Drawing for the job (mm, zero at the part's lowest x, y, z). A direction names the side the tool comes from. Coordinates: 2 decimals unless noted, no trailing zeros. Order: outer loops, then holes, each group sorted by start corner. A loop starts at its lowest first (then second) coordinate and runs counter-clockwise, first axis right, second up. Notation, with made-up numbers: (-33.5, 32) - (1.5, 32) arc R33 ccw to (1.5, 67) - close; hole circle Ø4 at (-37.5, 26). An arc over 180 degrees is marked (long way). Put each result on its own line as item: value. Start each with the question number.
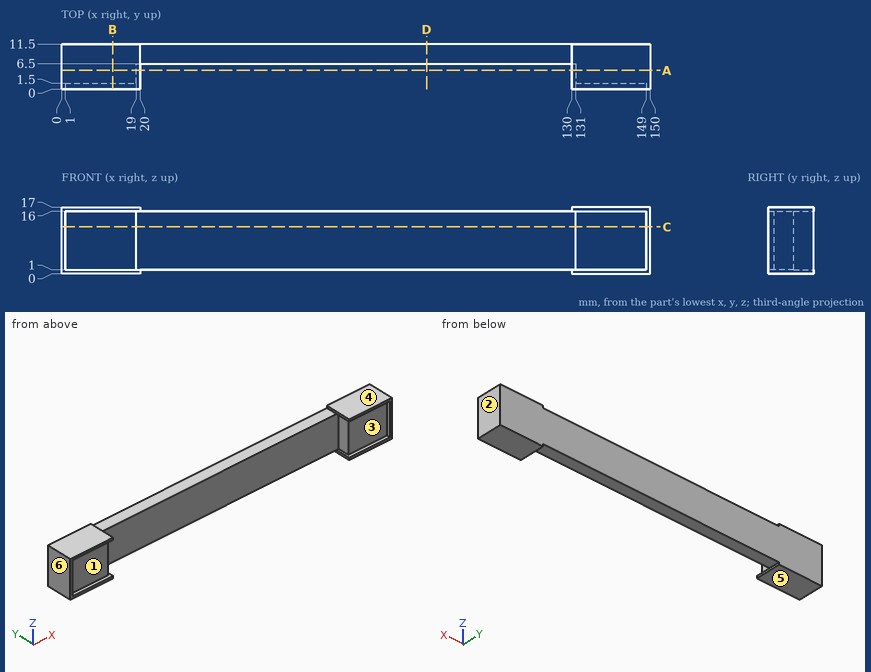
Item 1: Slice it at B-B, the plane x = 13. Give the cut face in (y, z), plus the area to 3 significant figures.
Item 2: Pull direction Z, two halves, no side cores. Call the marked faces 3, 4, 5 and 6: pulls with the +Z half, pulls with the -Z half, needs draft (parallel to the pull), parting line crosses it, or undercut.
Item 3: Flat gauge pins, fed straight in: pin 1 Ø1.2 at (y, z) = (1, 9.5) entering from -X; pin 2 Ø1 at (x, z) = (41, 9.5) entering from -Y; pin 3 Ø4.5 at (x, z) = (136, 12) entering from -Y; pin 4 Ø5.5 at (x, y) = (90, 8.5) entering from +Z. Where does each tip first touch, or does it go through?
Item 4: Slice it at C-C, the plane z = 12. Give the cut face in (x, y), plus the area to 3 significant figures.
Item 5: Slice it at A-A, the plane y = 4.75. Give the cut face in (x, z).
Item 6: 3-axis set-ups, long thin cutter, end or side, ignore diameter. For the marked faces 1 and 2: which of +Z, -Z, +X, -X, +Y, -Y reach the whole face in a straight line?
Item 7: Wall check: line 1 along X through (y, z) = (1, 3.25); line 2 along X through (y, z) = (3, 7); line 3 along Z through (x, y) = (125, 10.5). Give the ranges that are in metal, low to high.
Item 8: Slice it at D-D, the plane x = 93. Give the cut face in (y, z).
Here are the results:
1. outline: (0, 0) - (11.5, 0) - (11.5, 17) - (0, 17) - (0, 16) - (1.5, 16) - (1.5, 1) - (0, 1) - close
1. area: 173 mm^2
2. face 3: undercut
2. face 4: pulls with the +Z half
2. face 5: pulls with the -Z half
2. face 6: needs draft
3. pin 1: stops at x = 0
3. pin 2: stops at y = 6.5
3. pin 3: stops at y = 1.5
3. pin 4: stops at z = 16
4. outline: (0, 0) - (1, 0) - (1, 1.5) - (19, 1.5) - (19, 6.5) - (131, 6.5) - (131, 1.5) - (149, 1.5) - (149, 0) - (150, 0) - (150, 11.5) - (0, 11.5) - close
4. area: 943 mm^2
5. outline: (0, 0) - (20, 0) - (20, 1) - (19, 1) - (19, 16) - (20, 16) - (20, 17) - (0, 17) - close; (130, 0) - (150, 0) - (150, 17) - (130, 17) - (130, 16) - (131, 16) - (131, 1) - (130, 1) - close
6. face 1: -Y
6. face 2: +Z, -Z, +X, +Y, -Y
7. line 1: x = 0 to 1, 149 to 150
7. line 2: x = 0 to 19, 131 to 150
7. line 3: z = 1 to 16
8. outline: (6.5, 1) - (11.5, 1) - (11.5, 16) - (6.5, 16) - close
